Geometry: final body of the model. Coordinates: model frame, mm. Face numbers are marked on the shaded views. A direction names the side the tool comes from. Give positions to 0.01 mm unless a question says otherwise; leave off trailing zeros. Order: outer loops, then holes, each group sorted by start corner. A loop starts at its lowest first (then second) coordinate and runs counter-clockwise, first axis right, second up. Notation, with made-up numbers: M -15,-37.5 L 37,-37.5 A12 ccw 37,-20.5 Z; hole C 7,51.5 d1. An arc over 180 degrees is marked long. One line per item, written item: value. Start each with the question number.
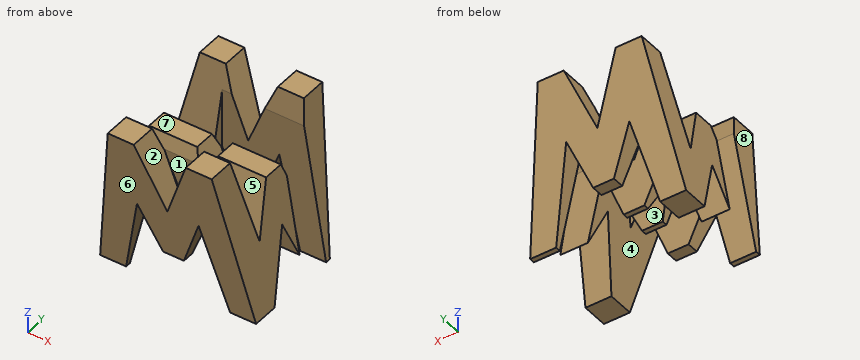
```python
from build123d import *

# Parameters (mm, degrees)
F0_W      = 38.1
F0_H      = 38.1
F1_DEPTH  = 38.1
F6_DEPTH  = 38.1
F8_DEPTH  = 38.1
F9_W      = 25.4
F9_H      = 7.62
F10_DEPTH = 38.1


with BuildPart() as f1:
    # F0 (on Front) → F1 (new body)
    with BuildSketch(Plane.XZ):
        with Locations((19.05, 19.05)):
            Rectangle(F0_W, F0_H)
    extrude(amount=F1_DEPTH)

    # F5 (on offset) → F6 (cut)
    with BuildSketch(Plane.YZ.offset(38.1)):
        Polygon((-31.75, 0), (-38.1, 38.1), (-38.1, 0), align=None)
        Polygon((-11.43, 14.970142), (-6.35, 38.1), (-31.75, 38.1), (-26.67, 16.447108), (-21.59, 28.575), (-16.51, 28.575), align=None)
        Polygon((-25.4, 0), (-12.7, 0), (-19.05, 15.875), align=None)
        Polygon((-6.35, 0), (0, 0), (0, 38.1), align=None)
    extrude(amount=-F6_DEPTH, mode=Mode.SUBTRACT)

    # F7 (on offset) → F8 (cut)
    with BuildSketch(Plane.XZ.offset(38.1)):
        Polygon((0, 38.1), (0, 0), (6.35, 38.1), align=None)
        Polygon((25.4, 38.1), (12.7, 38.1), (19.05, 22.225), align=None)
        Polygon((11.43, 20.620601), (6.35, 0), (31.75, 0), (26.67, 22.225), (21.59, 9.525), (16.51, 9.525), align=None)
        Polygon((31.75, 38.1), (38.1, 0), (38.1, 38.1), align=None)
    extrude(amount=-F8_DEPTH, mode=Mode.SUBTRACT)

    # F9 (on offset) → F10 (cut)
    with BuildSketch(Plane.XY.offset(38.1)):
        with Locations((25.4, -11.43)):
            Rectangle(F9_W, F9_H)
        with Locations((12.7, -26.67)):
            Rectangle(F9_W, F9_H)
    extrude(amount=-F10_DEPTH, mode=Mode.SUBTRACT)


solid = f1.part
```
Q1. Section query C-C on z = 31. Return loops of the section in (x, y), and give its area (3 significant figures).
Q2. Section query A-A on z = 4. Return loops of the section in (x, y), and give its area (3 significant figures).
Q3. Contact query for flat-ended pins moving along their axis: pin 1 (3.5 mm diameter, centred on y = -9.5, z = 25, fed in from +X); pin 2 (1.5 mm diameter, centred on y = -34, z = 33, fed in from +X) (3 decimals); pin 3 (10 mm diameter, centred on y = -17, z = 23.5, fed in from +X). Output: stop coordinate, or through.
Q4. Mould query, pull axis Y, two halves, no side actions, for the marked faces 6, 7 and 8. Classes: +Y half, -Y half, draft (parallel to the pull), parting line (faces both ways), or undercut.
Q5. Ray query, line 1 along Y through (x, z) = (23.5, 28.5); line 2 along Y through (x, z) = (14.5, 20); line 3 along X through (y, z) = (-7, 13). Return the intervals inside material, ascending. Write a range as [from, to].
Q6. Set-up query: the marked faces 1, 2, 3, 4 and 5. Return all of +Z, -Z, +X, -X, +Y, -Y with unobstructed straight access to the full face (end or side cutting, diameter ignored); none if empty.
Results below:
1. outline: M 5.17,-36.92 L 15.54,-36.92 L 15.54,-30.48 L 5.17,-30.48 Z; M 5.17,-7.91 L 12.7,-7.91 L 12.7,-7.62 L 15.54,-7.62 L 15.54,-1.18 L 5.17,-1.18 Z; M 22.56,-36.92 L 32.93,-36.92 L 32.93,-30.08 L 25.4,-30.08 L 25.4,-30.48 L 22.56,-30.48 Z; M 22.56,-7.62 L 32.93,-7.62 L 32.93,-1.18 L 22.56,-1.18 Z
1. area: 272 mm2
2. outline: M 0.67,-32.42 L 7.34,-32.42 L 7.34,-30.48 L 0.67,-30.48 Z; M 0.67,-14.3 L 7.34,-14.3 L 7.34,-5.68 L 0.67,-5.68 Z; M 30.84,-32.42 L 37.43,-32.42 L 37.43,-23.8 L 30.84,-23.8 Z; M 30.84,-7.62 L 37.43,-7.62 L 37.43,-5.68 L 30.84,-5.68 Z
2. area: 140 mm2
3. pin 1: x = 12.7
3. pin 2: x = 32.725
3. pin 3: x = 35.02
4. face 6: -Y half
4. face 7: undercut
4. face 8: draft
5. line 1: [-36.5, -30.48], [-21.62, -16.48], [-7.62, -1.6]
5. line 2: [-35.08, -30.48], [-22.86, -15.24], [-7.62, -3.02]
5. line 3: [2.17, 9.55], [14.92, 22.98], [28.78, 35.93]
6. face 1: +Z, -Z, -X
6. face 2: +Z, +Y, -Y
6. face 3: -Z, +X, -X
6. face 4: -Z, +Y, -Y
6. face 5: +Z, +X, -X
